Can you work these out from the model? Positions are in its coordinate system, mm. A direction names the side the tool comes from. Give positions to 0.01 mm unless a question says otherwise; leave off trailing zeros. Order: outer loops, then holes, each group sorted by start corner. A loop starts at its lowest first (then second) coordinate and runs counter-clockwise, first axis right, second up. Notation, with made-up numbers: (32.25, -34.5) - (72.25, -34.5) arc R22 cw to (72.25, -14.5) - close; hole circle Ø11 at (1, 2). An arc over 180 degrees is marked (long way). Use one line per item in the form item = value. Start each with the question number.
1) Suppose I cut it at A-A, the plane x = -2. Write out the boundary of the cut face in (y, z), and give its area (3 significant figures).
2) Which directions (+Z, -Z, +X, -X, +Y, -Y) give clear straight access to the entire face, cutting with the end or side of a thin tool? Please do faces 4 (the flat face through (-6, -27, 15)), 5 (the flat face through (-3, -25.829, 4)).
3) Suppose I cut it at D-D, the plane z = -1.75. Write out the boundary of the cut face in (x, y), and give its area (3 significant figures).
4) We'd pull the mould along Y, two halves only. Please class faces 1 (the flat face through (-3, -42.729, 4)), 2 (the flat face through (-6, -27, -7)), 3 (the flat face through (-6, -59.779, 4)): released by +Y, released by -Y, zero draft, split by the parting line, or undercut.
5) Suppose I cut it at C-C, the plane x = -7. Write out the boundary of the cut face in (y, z).
6) Please list where these lines run through material, in increasing order: probe 1 along Y at (x, z) = (-3.5, 4); probe 2 along Z at (x, y) = (-6.25, -33.5); probe 3 along Y at (x, z) = (-0.5, 8.75).
7) Suppose I cut it at B-B, the plane z = 4. Write out the boundary of the cut face in (x, y), and give its area (3 significant figures).
```python
from build123d import *

# Parameters (mm, degrees)
SKETCH_1_W          = 23
SKETCH_1_H          = 64.4
EXTRUDE_1_DEPTH     = 8
SKETCH_3_W          = 23
SKETCH_3_H          = 64.4
SKETCH_3_R          = 5.5
EXTRUDE_2_DEPTH     = 7
SKETCH_4_W          = 23
SKETCH_4_H          = 64.4
SKETCH_4_R          = 5.5
EXTRUDE_3_DEPTH     = 7
SKETCH_5_R          = 1.65
CUT_EXTRUDE_1_DEPTH = 24
SKETCH_6_W          = 22
SKETCH_6_H          = 64.4
CUT_EXTRUDE_2_DEPTH = 11


with BuildPart() as part:
    # 草圖1 → 填料-伸長1 (new body)
    with BuildSketch(Plane.XY):
        with Locations((-0.36746988, -27.579314659)):
            Rectangle(SKETCH_1_W, SKETCH_1_H)
        Polygon((9.38974967, -34.279314659), (4.511139895, -25.829314659), (-5.246079654, -25.829314659), (-10.124689429, -34.279314659), (-5.246079654, -42.729314659), (4.511139895, -42.729314659), align=None, mode=Mode.SUBTRACT)
    extrude(amount=EXTRUDE_1_DEPTH)

    # 草圖3 → 填料-伸長2 (add)
    with BuildSketch(Plane.XY.offset(8)):
        with Locations((-0.36746988, -27.579314659)):
            Rectangle(SKETCH_3_W, SKETCH_3_H)
        with Locations((-0.36746988, -34.279314659)):
            Circle(SKETCH_3_R, mode=Mode.SUBTRACT)
    extrude(amount=EXTRUDE_2_DEPTH)

    # 草圖4 → 填料-伸長3 (add)
    with BuildSketch(Plane(origin=(0, 0, 0), x_dir=(-1, 0, 0), z_dir=(0, 0, -1))):
        with Locations((0.36746988, -27.579314659)):
            Rectangle(SKETCH_4_W, SKETCH_4_H)
        with Locations((0.36746988, -34.279314659)):
            Circle(SKETCH_4_R, mode=Mode.SUBTRACT)
    extrude(amount=EXTRUDE_3_DEPTH)

    # 草圖5 → 除料-伸長1 (cut, through all)
    with BuildSketch(Plane(origin=(11.13253012, 0, 0), x_dir=(0, 0, -1), z_dir=(1, 0, 0))):
        with Locations((-4, -7.779314659)):
            Circle(SKETCH_5_R)
    extrude(amount=-CUT_EXTRUDE_1_DEPTH, mode=Mode.SUBTRACT)

    # 草圖6 → 除料-伸長2 (cut)
    with BuildSketch(Plane(origin=(11.13253012, 0, 0), x_dir=(0, 0, -1), z_dir=(1, 0, 0))):
        with Locations((-4, -27.579314659)):
            Rectangle(SKETCH_6_W, SKETCH_6_H)
    extrude(amount=-CUT_EXTRUDE_2_DEPTH, mode=Mode.SUBTRACT)


solid = part.part
```
Result sheet:
q1.outline = (-59.78, -7) - (-39.53, -7) - (-39.53, 0) - (-42.73, 0) - (-42.73, 8) - (-39.53, 8) - (-39.53, 15) - (-59.78, 15) - close; (-29.03, -7) - (4.62, -7) - (4.62, 15) - (-29.03, 15) - (-29.03, 8) - (-25.83, 8) - (-25.83, 0) - (-29.03, 0) - close; hole circle Ø3.3 at (-7.78, 4)
q1.area = 1,130 mm²
q2.face_4 = +Z, +X, -X, +Y, -Y
q2.face_5 = +X
q3.outline = (-11.87, -59.78) - (0.13, -59.78) - (0.13, -39.76) arc R5.5 cw (long way) to (0.13, -28.8) - (0.13, 4.62) - (-11.87, 4.62) - close
q3.area = 720 mm²
q4.face_1 = undercut
q4.face_2 = zero draft
q4.face_3 = released by -Y
q5.outline = (-59.78, -7) - (4.62, -7) - (4.62, 15) - (-59.78, 15) - close; hole (-39.69, 0) - (-28.87, 0) - (-28.87, 8) - (-39.69, 8) - close; hole circle Ø3.3 at (-7.78, 4)
q6.probe_1 = -59.78 to -42.73, -25.83 to -9.43, -6.13 to 4.62
q6.probe_2 = -7 to 0, 8 to 15
q6.probe_3 = -59.78 to -39.78, -28.78 to 4.62
q7.outline = (-11.87, -59.78) - (0.13, -59.78) - (0.13, -42.73) - (-5.25, -42.73) - (-10.12, -34.28) - (-5.25, -25.83) - (0.13, -25.83) - (0.13, -9.43) - (-11.87, -9.43) - close; (-11.87, -6.13) - (0.13, -6.13) - (0.13, 4.62) - (-11.87, 4.62) - close
q7.area = 601 mm²
